Source: CAD feature listing. Evaluate the final solid. Frame: model axes, mm. Face numbers are marked on the shaded views. A direction names the side the tool comes from. Coordinates: 2 decimals unless noted, no trailing zeros. Order: outer loops, then holes, each group sorted by start corner. A loop starts at its lowest first (then second) coordinate and runs counter-clockwise, first axis right, second up. Notation, with made-up numbers: (21.25, 32) - (68.25, 32) arc R14 cw to (68.25, 48) - close; hole circle Ø3 at (15, 52.25). An arc over 180 degrees is marked (long way). One line per question, with ' | ' between items. Start each with the question number.
(1) Line query: line 1 along Z through (x, y) = (0, -3.3); line 2 along Y through (x, z) = (7.75, 0); line 3 along Y through (x, z) = (1.75, -1). Output: solid intervals per line, ascending.
(2) Section C-C (y = 1). Return the cut outline in (x, z), then the cut area to 3 significant figures.
(3) Contact query for flat-ended pins moving along their axis: P1, Ø5.5, axis at x = 0, z = 0, coming from the -Y side; P2, Ø8, axis at x = 5, z = -0.5, coming from the -Y side; P3, Ø1.5, axis at y = 2.5, z = 3, coming from the +X side; P4, Ø4, axis at x = -5, y = 0, coming from the -Z side. Output: stop coordinate, or through.
(4) Section B-B (x = 6). Return the cut outline in (y, z).
(5) Section D-D (z = 5.5). Return the cut outline in (x, y).
(6) Access query for the marked faces 1, 2 and 3. Directions: +Z, -Z, +X, -X, +Y, -Y. A direction counts if a zero-diameter tool reaches every point of the face in a straight line with its end or side. Return the directions, or none.
(7) Section A-A (z = 0). Return the cut outline in (x, y).
(8) Draft query along Z for the marked faces 4, 5 and 6. Return one class per face: +Z half, -Z half, draft (parallel to the pull), parting line (faces both ways), or undercut.
Autodesk Inventor part; units mm, degrees
ref_plane "YZ Plane" through (0, 0, 0) normal (1, 0, 0) x (0, 1, 0)
ref_plane "XZ Plane" through (0, 0, 0) normal (0, 1, 0) x (-1, 0, 0)
ref_plane "XY Plane" through (0, 0, 0) normal (0, 0, 1) x (1, 0, 0)
sketch "Boceto1" plane through (0, 0, 0) normal (0, 1, 0) x (-1, 0, 0)
  circle A0 centre (0, 0) radius 8.1
  dimension "d0" = 16.2
extrude "Extrusión1" add sketch "Boceto1" along normal blind 1.3
sketch "Boceto2" plane through (0, 1.3, 0) normal (0, 1, 0) x (1, 0, 0)
  circle A0 centre (0, 0) radius 4.55
  dimension "d3" = 9.1
extrude "Extrusión2" add sketch "Boceto2" along normal blind 3.3
sketch "Boceto3" plane through (0, 4.6, 0) normal (0, 1, 0) x (1, 0, 0)
  circle A0 centre (0, 0) radius 3.1
  dimension "d6" = 6.2
extrude "Extrusión3" cut sketch "Boceto3" against normal blind 3.2
sketch "Boceto4" plane through (0, 1.4, 0) normal (0, 1, 0) x (1, 0, 0)
  arc A0 (0, -1.5) -> (0, 1.5) centre (0, 0) ccw
  line L0 (0, -1.5) -> (-7.9599, -1.5)
  circle A1 centre (0, 0) radius 8.1
  line L1 (0, 1.5) -> (-7.9599, 1.5)
  arc A2 (-7.9599, 1.5) -> (-7.9599, -1.5) centre (0, 0) ccw
  dimension "d9" = 3
extrude "Extrusión4" cut sketch "Boceto4" along normal blind 3.2 and the other way blind 1.6 contours L0 A1 L1 A0 picked at (-2.6948, -0.1675)
fillet "Empalme1" radius 0.3 1 edges at (4.55, 1.3, 0)
sketch "Boceto5" plane through (0, 0, 0) normal (0, -1, 0) x (1, 0, 0)
  arc A0 (-6.4786, -1.5) -> (-6.4786, 1.5) centre (0, 0) ccw
  arc A1 (-5.5509, -1.5) -> (-5.5509, 1.5) centre (0, 0) ccw
  line L0 (-7.9599, 1.5) -> (0, 1.5)
  line L1 (-5.5509, 1.5) -> (-6.4786, 1.5)
  line L2 (-7.9599, -1.5) -> (-4.6122, -1.5)
  line L3 (-6.4786, -1.5) -> (-5.5509, -1.5)
  dimension "d15" = 13.3
  dimension "d16" = 11.5
extrude "Extrusión5" add sketch "Boceto5" along normal blind 4.3
properties part number "Pieza_Presion_resorte" material "Plástico ABS"
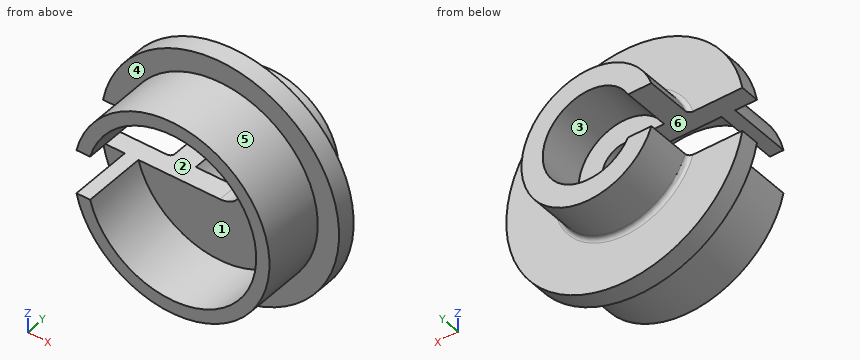
Response values:
1) line 1: z = -6.65 to -5.75, 5.75 to 6.65 | line 2: y = 0 to 1.3 | line 3: y = 0 to 1.4
2) outline: (-7.96, -1.5) arc R8.1 ccw (long way) to (-7.96, 1.5) - (0, 1.5) arc R1.5 cw to (0, -1.5) - close | area: 178 mm²
3) P1: stops at y = 0 | P2: stops at y = -4.3 | P3: stops at x = 3.95 | P4: stops at z = -7.52
4) outline: (-4.3, -2.87) - (0, -2.87) - (0, -5.44) - (1.3, -5.44) - (1.3, 5.44) - (0, 5.44) - (0, 2.87) - (-4.3, 2.87) - close
5) outline: (-5.95, 0) - (-3.74, 0) - (-3.74, -4.3) - (-1.68, -4.3) - (-1.68, 0) - (1.68, 0) - (1.68, -4.3) - (3.74, -4.3) - (3.74, 0) - (5.95, 0) - (5.95, 1.3) - (-5.95, 1.3) - close
6) face 1: -Y | face 2: -X, +Y, -Y | face 3: +Y
7) outline: (1.5, 0) - (5.75, 0) - (5.75, -4.3) - (6.65, -4.3) - (6.65, 0) - (8.1, 0) - (8.1, 1.3) - (4.85, 1.3) arc R0.3 cw to (4.55, 1.6) - (4.55, 4.6) - (3.1, 4.6) - (3.1, 1.4) - (1.5, 1.4) - close
8) face 4: draft | face 5: parting line | face 6: undercut
